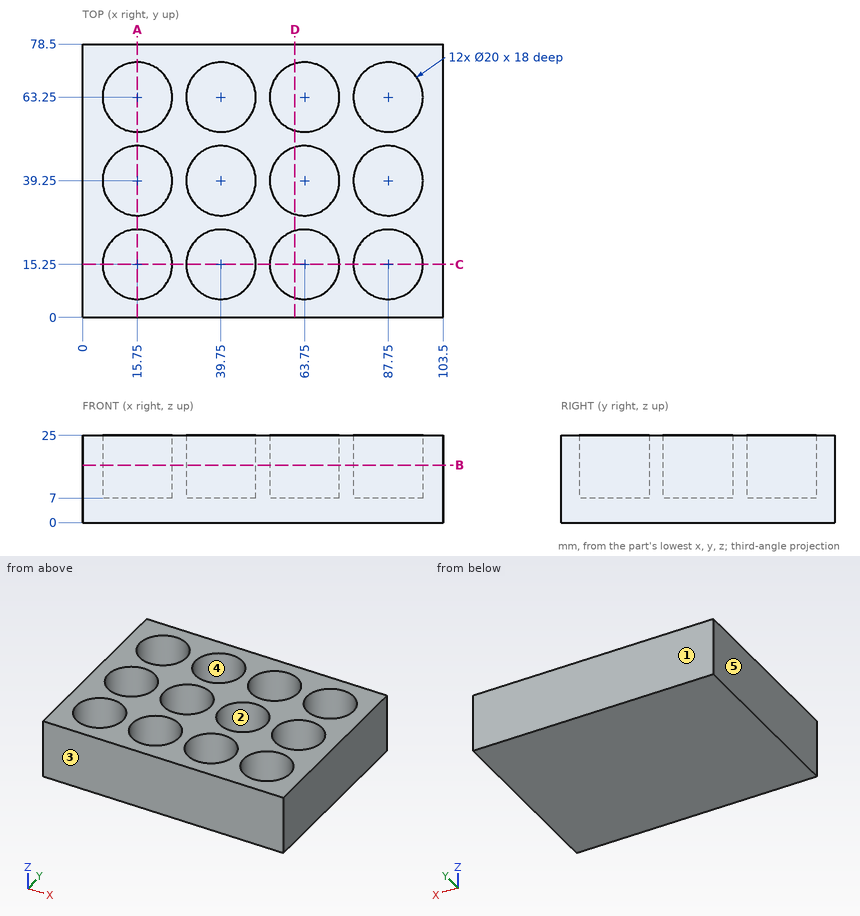
Can you work these out from the drawing? Everything is in mm from the part's minimum corner. A direction names the side the tool comes from. Coordinates: 2 decimals unless noted, no trailing zeros. Write each loop counter-clockwise with the first axis right and the second up, starting at its lowest first coordinate (ties: lowest second). Pieces come first, ordered by that corner, then holes. Notation, with made-up numbers: (11.5, -31.75) - (39.5, -31.75) arc R11 ccw to (39.5, -21.75) - close; hole circle Ø4 at (11.25, -36.5). An arc over 180 degrees is marked (long way). Use a Markdown table: item, result.
Q1. Imagine slicing it at D-D (x = 61). List the corners of the cut face in (y, z) for me.
Geometry check:
| item | result |
|---|---|
| outline | (0, 0) - (78.5, 0) - (78.5, 25) - (72.86, 25) - (72.86, 7) - (53.64, 7) - (53.64, 25) - (48.86, 25) - (48.86, 7) - (29.64, 7) - (29.64, 25) - (24.86, 25) - (24.86, 7) - (5.64, 7) - (5.64, 25) - (0, 25) - close |
Q2. Imagine slicing it at C-C (y = 15.25). List the corners of the cut face in (x, z) for me.
Geometry check:
| item | result |
|---|---|
| outline | (0, 0) - (103.5, 0) - (103.5, 25) - (97.75, 25) - (97.75, 7) - (77.75, 7) - (77.75, 25) - (73.75, 25) - (73.75, 7) - (53.75, 7) - (53.75, 25) - (49.75, 25) - (49.75, 7) - (29.75, 7) - (29.75, 25) - (25.75, 25) - (25.75, 7) - (5.75, 7) - (5.75, 25) - (0, 25) - close |
Q3. I'm going to push a flat-ended pin straight in: pin 1 Ø16 at (x, y) = (15.75, 63.25) entering from +Z. Where does the tip first touch, or does it pass through?
Geometry check:
| item | result |
|---|---|
| pin 1 | stops at z = 7 |
Q4. Please list where these lines run through material, in increasing order: L1, parallel to Y at x = 87.75, z = 11.5; L2, parallel to X at y = 63, z = 21; L3, parallel to Y at x = 60, z = 23.75.
Geometry check:
| item | result |
|---|---|
| L1 | y = 0 to 5.25, 25.25 to 29.25, 49.25 to 53.25, 73.25 to 78.5 |
| L2 | x = 0 to 5.75, 25.75 to 29.75, 49.75 to 53.75, 73.75 to 77.75, 97.75 to 103.5 |
| L3 | y = 0 to 5.98, 24.52 to 29.98, 48.52 to 53.98, 72.52 to 78.5 |
Q5. Imagine slicing it at B-B (z = 16.5). Count the separate pieces of the cut face and the enclosed holes in it, and give its area (3 significant figures).
Geometry check:
| item | result |
|---|---|
| separate pieces | 1 |
| enclosed holes | 12 |
| area | 4,350 mm2 |
Q6. Thinking about a two-plate mould opening in Y: for the marked faces 3, 4 and 5, which applies, +Y half, -Y half, draft (parallel to the pull), parting line (faces both ways), or undercut?
Geometry check:
| item | result |
|---|---|
| face 3 | -Y half |
| face 4 | undercut |
| face 5 | draft |
Q7. Imagine slicing it at A-A (x = 15.75). List the corners of the cut face in (y, z) for me.
Geometry check:
| item | result |
|---|---|
| outline | (0, 0) - (78.5, 0) - (78.5, 25) - (73.25, 25) - (73.25, 7) - (53.25, 7) - (53.25, 25) - (49.25, 25) - (49.25, 7) - (29.25, 7) - (29.25, 25) - (25.25, 25) - (25.25, 7) - (5.25, 7) - (5.25, 25) - (0, 25) - close |
Q8. Which directions (+Z, -Z, +X, -X, +Y, -Y) give clear straight access to the entire face, cutting with the end or side of a thin tool? Please do the marked faces 1 and 2.
Geometry check:
| item | result |
|---|---|
| face 1 | +Z, -Z, +X, -X, +Y |
| face 2 | +Z |
